Read the model definition and answer for the solid it produces. Units are mm, in the model's axes. Face numbers are marked on the shaded views. A direction names the side the tool comes from. Round coordinates to 2 decimals unless told otherwise and drop trailing zeros. Write each loop counter-clockwise with the first axis right and the second up, starting at its lowest first coordinate (ties: lowest second). Pieces come first, ordered by that corner, then holes.
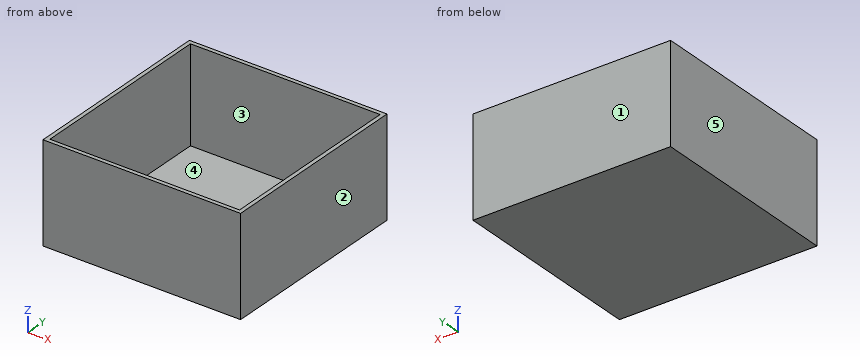
from build123d import *

# Parameters (mm, degrees)
F0_W          = 127
F0_H          = 63.5
F1_DEPTH      = 63.5
F1_DEPTH_BACK = 63.5
F2_T          = -2.54


with BuildPart() as f1:
    # F0 (on Front) → F1 (new body, two sides)
    with BuildSketch(Plane.XZ) as f1_sk:
        with Locations((0, 31.75)):
            Rectangle(F0_W, F0_H)
    extrude(amount=F1_DEPTH)
    extrude(f1_sk.sketch, amount=-F1_DEPTH_BACK)

    # F2
    f2_openings = [f1.faces().sort_by_distance(p)[0] for p in [
        (0, 0, 63.5),
    ]]
    offset(amount=F2_T, openings=f2_openings)


solid = f1.part
Q1. Which of the six approach directions +Z, -Z, +X, -X, +Y, -Y give full straight-line access (tool end or side, diameter ignored) to the marked faces 4 and 5?
Verdict:
face 4: +Z
face 5: +Z, -Z, -X, +Y, -Y
Q2. Straight lines are drawn through the part: probe 1 along Y at (x, z) = (40, 6.5); probe 2 along Z at (x, y) = (-33, -53.5). For each, find the intervals that lie inside material, in ascending order.
Verdict:
probe 1: y = -63.5 to -60.96, 60.96 to 63.5
probe 2: z = 0 to 2.54
Q3. A flat-ended cylindrical pin translates along its axis: pin 1 Ø12 at (x, y) = (-33.5, 38) entering from +Z. Find the tip coordinate at first contact, or state that the pin passes through.
Verdict:
pin 1: stops at z = 2.54
Q4. Section A-A (z = 9) is taken. Determine the outline of the cut face in (x, y).
Verdict:
outline: (-63.5, -63.5) - (63.5, -63.5) - (63.5, 63.5) - (-63.5, 63.5) - close; hole (-60.96, -60.96) - (60.96, -60.96) - (60.96, 60.96) - (-60.96, 60.96) - close
Q5. Section B-B (y = 50) is taken. Determine the outline of the cut face in (x, z), then the cut area to 3 significant figures.
Verdict:
outline: (-63.5, 0) - (63.5, 0) - (63.5, 63.5) - (60.96, 63.5) - (60.96, 2.54) - (-60.96, 2.54) - (-60.96, 63.5) - (-63.5, 63.5) - close
area: 632 mm2
Q6. Determine the mould class of the marked faces 1, 2 and 3 for opening direction Y: pulls with the +Y half, pulls with the -Y half, needs draft (parallel to the pull), parting line crosses it, or undercut.
Verdict:
face 1: pulls with the +Y half
face 2: needs draft
face 3: undercut
